from build123d import *

# Parameters (mm, degrees)
F1_DEPTH = 50.8
F3_R     = 3.175
F4_DEPTH = 177.801


with BuildPart() as f1:
    # F0 (on Front) → F1 (new body)
    with BuildSketch(Plane.XZ):
        Polygon((25.4, 177.8), (0, 0), (6.414469, 0), (30.000183, 165.1), (198.599817, 165.1), (222.185531, 0), (228.6, 0), (203.2, 177.8), align=None)
    extrude(amount=F1_DEPTH)


with BuildPart() as f1_1:
    # F2: moved
    add(f1.part.moved(Location((-114.3, 0, 0))))

    # F3 (on face) → F4 (cut, through all)
    with BuildSketch(Plane.XY.offset(177.8)):
        with Locations((-79.375, -6.35)):
            Circle(F3_R)
        with Locations((-79.375, -44.45)):
            Circle(F3_R)
        with Locations((79.375, -6.35)):
            Circle(F3_R)
        with Locations((79.375, -44.45)):
            Circle(F3_R)
    extrude(amount=-F4_DEPTH, mode=Mode.SUBTRACT)


solid = f1_1.part
Input: part model. Units: mm. Frame: model coordinates. A direction names the side the tool comes from. Round coordinates to 2 decimals unless told otherwise and drop trailing zeros. Order: outer loops, then holes, each group sorted by start corner. A loop starts at its lowest first (then second) coordinate and runs counter-clockwise, first axis right, second up. Notation, with made-up numbers: (-28, 75) - (14, 75) arc R32 cw to (14, 109) - close; hole circle Ø2 at (-8.75, -30). An arc over 180 degrees is marked (long way). Use a Markdown table: item, result.
1. Mould query, pull axis X, two halves, no side actions, for faces 1 (the face through (-1, -25, 165.1)), 2 (the face through (101.778, -25.044, 87.655)), 3 (the face through (111, -25, 0)). Classes: +X half, -X half, draft (parallel to the pull), parting line (faces both ways), or undercut.
Evaluation:
| item | result |
|---|---|
| face 1 | undercut |
| face 2 | +X half |
| face 3 | draft |
2. Access query for faces 4 (the face through (95.928, -25.044, 83.706)), 5 (the face through (-76.347, -43.496, 171.539)). Directions: +Z, -Z, +X, -X, +Y, -Y. A direction counts if a zero-diameter tool reaches every point of the face in a straight line with its end or side. Return the directions, or none.
Evaluation:
| item | result |
|---|---|
| face 4 | -Z, +Y, -Y |
| face 5 | +Z, -Z |
3. Section D-D on z = 61. Return the cut outline in (x, y).
Evaluation:
| item | result |
|---|---|
| outline | (-105.59, -50.8) - (-99.17, -50.8) - (-99.17, 0) - (-105.59, 0) - close; (99.17, -50.8) - (105.59, -50.8) - (105.59, 0) - (99.17, 0) - close |
4. Section B-B on y = -18.5. Return the cut outline in (x, z), then the cut area to 3 significant figures.
Evaluation:
| item | result |
|---|---|
| outline | (-114.3, 0) - (-107.89, 0) - (-84.3, 165.1) - (84.3, 165.1) - (107.89, 0) - (114.3, 0) - (88.9, 177.8) - (-88.9, 177.8) - close |
| area | 4,400 mm^2 |
5. Section A-A on y = -6.35. Return the cut outline in (x, z).
Evaluation:
| item | result |
|---|---|
| outline | (-114.3, 0) - (-107.89, 0) - (-84.3, 165.1) - (-82.55, 165.1) - (-82.55, 177.8) - (-88.9, 177.8) - close; (-76.2, 165.1) - (76.2, 165.1) - (76.2, 177.8) - (-76.2, 177.8) - close; (82.55, 165.1) - (84.3, 165.1) - (107.89, 0) - (114.3, 0) - (88.9, 177.8) - (82.55, 177.8) - close |
6. Material intervals for probe 1 along X at (y, z) = (-6, 174); probe 2 along Z at (x, y) = (66, -8); probe 3 along X at (y, z) = (-36.5, 80.5), sorted ascending.
Evaluation:
| item | result |
|---|---|
| probe 1 | -89.44 to -82.53, -76.22 to 76.22, 82.53 to 89.44 |
| probe 2 | 165.1 to 177.8 |
| probe 3 | -102.8 to -96.39, 96.39 to 102.8 |
7. First-contact query: pin 1 (4 mm diameter, centred on x = -79.375, y = -44.45, fed in from +Z); pin 2 (8 mm diameter, centred on x = -61.5, y = -30, fed in from -Z); pin 3 (2 mm diameter, centred on y = -38.5, z = 137.5, fed in from +X); pin 4 (3 mm diameter, centred on y = -36, z = 118.5, fed in from -X). Flat tips, straight axial feed; report the tip coordinate or a pass-through.
Evaluation:
| item | result |
|---|---|
| pin 1 | through |
| pin 2 | z = 165.1 |
| pin 3 | x = 94.8 |
| pin 4 | x = -97.59 |
8. Section C-C on z = 167.5. Return the cut outline in (x, y) (3 decimals), then the cut area to 3 significant figures.
Evaluation:
| item | result |
|---|---|
| outline | (-90.371, -50.8) - (90.371, -50.8) - (90.371, 0) - (-90.371, 0) - close; hole circle Ø6.35 at (-79.375, -44.45); hole circle Ø6.35 at (-79.375, -6.35); hole circle Ø6.35 at (79.375, -44.45); hole circle Ø6.35 at (79.375, -6.35) |
| area | 9,060 mm^2 |
